Read the model definition and answer for the solid it produces. Units are mm, in the model's axes. A direction names the side the tool comes from. Round coordinates to 2 decimals unless told otherwise and drop trailing zeros. Order: outer loops, then holes, each group sorted by start corner. A loop starts at its lowest first (then second) coordinate and runs counter-clockwise, first axis right, second up. Notation, with made-up numbers: M 56.25,10.5 L 97.25,10.5 A13 cw 97.25,16.5 Z; hole C 36.5,53.5 d10. An arc over 180 degrees is marked long. Use one line per item in the form item = value. Start each with the question number.
from build123d import *

# Parameters (mm, degrees)
SKETCH_R              = 23
SKETCH_R_2            = 2.75
SKETCH_R_3            = 2
PAD_DEPTH             = 1
SKETCH001_R           = 1.65
POCKET_DEPTH          = 1415.215977
POLARPATTERN_COUNT    = 3
POCKET001_DEPTH       = 5
SKETCH003_R           = 1.1
SKETCH003_R_2         = 1.45
POCKET002_DEPTH       = 1.001
SKETCH004_R           = 1.45
POCKET003_DEPTH       = 1.001
SKETCH005_R           = 2.1
POCKET004_DEPTH       = 1.001
SKETCH006_R           = 1.65
POCKET005_DEPTH       = 1415.215977
POLARPATTERN001_COUNT = 4
FILLET_R              = 15


with BuildPart() as part:
    # Sketch → Pad (new body)
    with BuildSketch(Plane.XY):
        Polygon((103.553391, 250), (-103.553391, 250), (-250, 103.553391), (-250, -103.553391), (-103.553391, -250), (103.553391, -250), (250, -103.553391), (250, 103.553391), align=None)
        Circle(SKETCH_R, mode=Mode.SUBTRACT)
        with Locations((150, 150)):
            Circle(SKETCH_R_2, mode=Mode.SUBTRACT)
        with Locations((-150, 150)):
            Circle(SKETCH_R_2, mode=Mode.SUBTRACT)
        with Locations((-150, -150)):
            Circle(SKETCH_R_2, mode=Mode.SUBTRACT)
        with Locations((150, -150)):
            Circle(SKETCH_R_2, mode=Mode.SUBTRACT)
        with Locations((28.284271, 28.284271)):
            Circle(SKETCH_R_3, mode=Mode.SUBTRACT)
        with Locations((-28.284271, 28.284271)):
            Circle(SKETCH_R_3, mode=Mode.SUBTRACT)
        with Locations((-28.284271, -28.284271)):
            Circle(SKETCH_R_3, mode=Mode.SUBTRACT)
        with Locations((28.284271, -28.284271)):
            Circle(SKETCH_R_3, mode=Mode.SUBTRACT)
    extrude(amount=PAD_DEPTH)

    # Sketch001 → Pocket (cut, through all)
    with BuildSketch(Plane.XY):
        with Locations((169.926455, -5)):
            Circle(SKETCH001_R)
        with Locations((169.926455, -18)):
            Circle(SKETCH001_R)
    pocket = extrude(amount=POCKET_DEPTH, mode=Mode.SUBTRACT)

    # PolarPattern: Pocket ×3 about axis
    polarpattern_axis = Axis((0, 0, 0), (0, 0, 1))
    for i in range(1, POLARPATTERN_COUNT):
        add(pocket.rotate(polarpattern_axis, i * 360 / POLARPATTERN_COUNT), mode=Mode.SUBTRACT)

    # Sketch002 → Pocket001 (cut)
    with BuildSketch(Plane.XY):
        with BuildLine():
            ThreePointArc((-60, 8), (-68, 0), (-60, -8))
            Line((-60, -8), (60, -8))
            ThreePointArc((60, -8), (68, 0), (60, 8))
            Line((-60, 8), (60, 8))
        make_face()
    extrude(amount=POCKET001_DEPTH, mode=Mode.SUBTRACT)

    # Sketch003 → Pocket002 (cut, through all)
    with BuildSketch(Plane.XY):
        with Locations((-80, 71)):
            Circle(SKETCH003_R)
        with Locations((-80, 26)):
            Circle(SKETCH003_R)
        with Locations((-80, -26)):
            Circle(SKETCH003_R)
        with Locations((-80, -71)):
            Circle(SKETCH003_R)
        with Locations((-80, 0)):
            Circle(SKETCH003_R_2)
        with Locations((80, 71)):
            Circle(SKETCH003_R)
        with Locations((80, 26)):
            Circle(SKETCH003_R)
        with Locations((80, 0)):
            Circle(SKETCH003_R_2)
        with Locations((80, -26)):
            Circle(SKETCH003_R)
        with Locations((80, -71)):
            Circle(SKETCH003_R)
        Polygon((-95, 51), (-105, 51), (-105, 45), (-103.5, 45), (-103.5, 49.5), (-95, 49.5), align=None)
        Polygon((-105, -45), (-95, -45), (-101.312029, -49.5), (-96, -49.5), (-96, -51), (-106, -51), (-99.687971, -46.5), (-105, -46.5), align=None)
        Polygon((105, -51), (95, -51), (101.312029, -46.5), (96, -46.5), (96, -45), (106, -45), (99.687971, -49.5), (105, -49.5), align=None)
        Polygon((95, 45), (105, 45), (105, 51), (103.5, 51), (103.5, 46.5), (95, 46.5), align=None)
    extrude(amount=POCKET002_DEPTH, mode=Mode.SUBTRACT)

    # Sketch004 → Pocket003 (cut, through all)
    with BuildSketch(Plane.XY):
        with Locations((-32.5, -56.291651)):
            Circle(SKETCH004_R)
        with Locations((32.5, -56.291651)):
            Circle(SKETCH004_R)
        with Locations((-32.5, 56.291651)):
            Circle(SKETCH004_R)
        with Locations((32.5, 56.291651)):
            Circle(SKETCH004_R)
    extrude(amount=POCKET003_DEPTH, mode=Mode.SUBTRACT)

    # Sketch005 → Pocket004 (cut, through all)
    with BuildSketch(Plane.XY):
        with Locations((135, 150)):
            Circle(SKETCH005_R)
        with Locations((165, 150)):
            Circle(SKETCH005_R)
        with Locations((-165, 150)):
            Circle(SKETCH005_R)
        with Locations((-135, 150)):
            Circle(SKETCH005_R)
        with Locations((-165, -150)):
            Circle(SKETCH005_R)
        with Locations((-135, -150)):
            Circle(SKETCH005_R)
        with Locations((135, -150)):
            Circle(SKETCH005_R)
        with Locations((165, -150)):
            Circle(SKETCH005_R)
    extrude(amount=POCKET004_DEPTH, mode=Mode.SUBTRACT)

    # Sketch006 → Pocket005 (cut, through all)
    with BuildSketch(Plane.XY):
        with Locations((-161.970876, -52.035422)):
            Circle(SKETCH006_R)
        with Locations((-157.524615, -64.251426)):
            Circle(SKETCH006_R)
    pocket005 = extrude(amount=POCKET005_DEPTH, mode=Mode.SUBTRACT)

    # PolarPattern001: Pocket005 ×4 about axis
    polarpattern001_axis = Axis((0, 0, 0), (0, 0, 1))
    for i in range(1, POLARPATTERN001_COUNT):
        add(pocket005.rotate(polarpattern001_axis, i * 360 / POLARPATTERN001_COUNT), mode=Mode.SUBTRACT)

    # Fillet
    fillet_edges = [part.edges().sort_by_distance(p)[0] for p in [
        (-250, -103.553391, 0.5),
        (-103.553391, -250, 0.5),
        (103.553391, -250, 0.5),
        (-250, 103.553391, 0.5),
        (-103.553391, 250, 0.5),
        (103.553391, 250, 0.5),
        (250, 103.553391, 0.5),
        (250, -103.553391, 0.5),
    ]]
    fillet(fillet_edges, radius=FILLET_R)


solid = part.part
Item 1: A tool of negligible diameter and unlimited length cuts with its end or side. For faces 4 (the cylindrical face through (0.391, 22.997, 0.493)), 5 (the flat face through (177.74, 175.813, 0.493)), from which of +Z, -Z, +X, -X, +Y, -Y can it reach the whole face along a straight path? Write none if from no direction.
Item 2: For a pull along Y with two mould halves and no side action, classify faces 1 (the cylindrical face through (-0.391, -22.997, 0.493)), 2 (the flat face through (-3, 59, 1)), 3 (the flat face through (-177.74, -175.813, 0.493)) as pulls with the +Y half, pulls with the -Y half, needs draft (parallel to the pull), parting line crosses it, or undercut.
Item 3: Section B-B (z = 0.75) is taken. Give the number of separate pieces and of enclosed holes in the cut face, and give its area (3 significant figures).
Item 4: Section C-C (y = 176.5) is taken. Write down the section's boundary in (x, z).
Item 5: Section A-A (x = 193) is taken. Write down the section's boundary in (y, z).
Item 6: Given P1, Ø4, axis at x = 165, y = -150, coming from the -Z side, flat-ended and moving along its own axis, determine where the tip first touches the part or whether it passes through.
Item 7: Find the intervals of material crossed by L1, parallel to Y at x = -32.5, z = 0.8; L2, parallel to Y at x = 135, z = 0.75; L3, parallel to Y at x = 169, z = 0.8, in increasing order. Write a range as [from, to].
The answers:
q1.face_4 = +Z, -Z
q1.face_5 = +Z, -Z, +X, +Y
q2.face_1 = undercut
q2.face_2 = needs draft
q2.face_3 = pulls with the -Y half
q3.separate_pieces = 1
q3.enclosed_holes = 49
q3.area = 203,000 mm²
q4.outline = M -177.05,0 L 177.05,0 L 177.05,1 L -177.05,1 Z
q5.outline = M -160.55,0 L 160.55,0 L 160.55,1 L -160.55,1 Z
q6.P1 = through
q7.L1 = [-250, -57.74], [-54.84, -8], [8, 54.84], [57.74, 250]
q7.L2 = [-218.55, -152.1], [-147.9, 147.9], [152.1, 218.55]
q7.L3 = [-184.55, -19.37], [-16.63, -6.37], [-3.63, 184.55]
